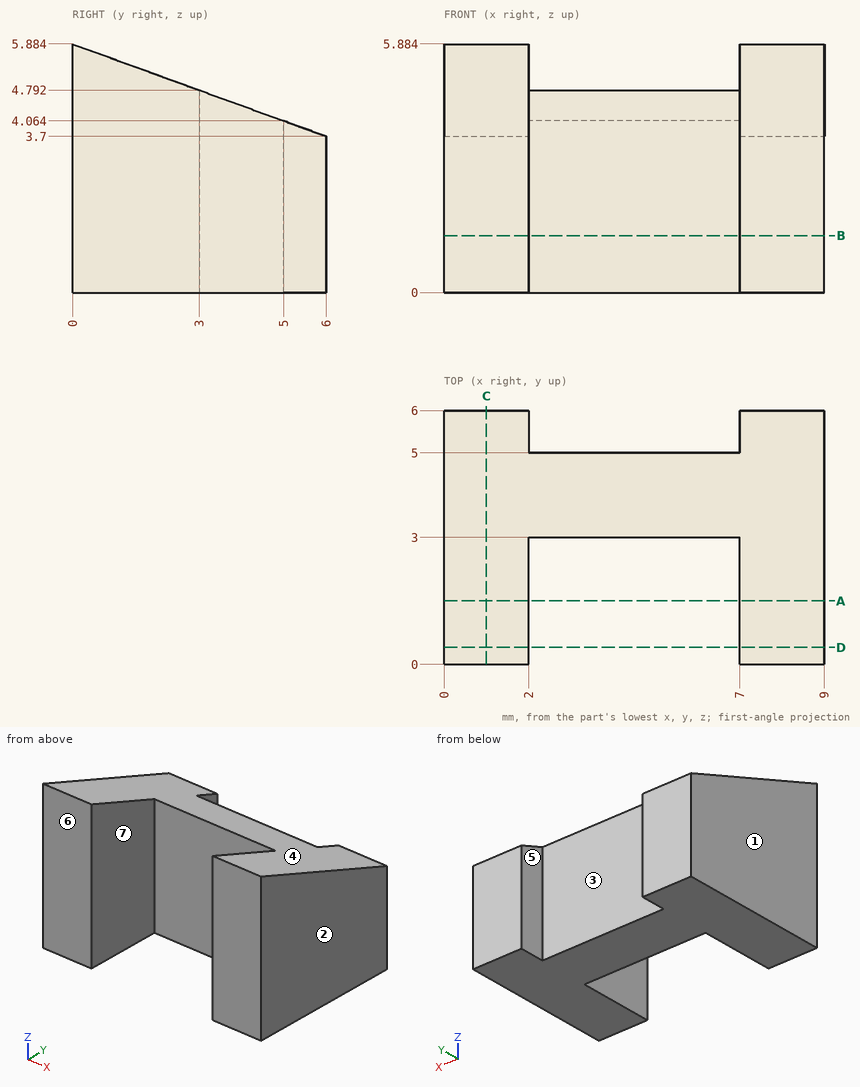
Answer from the drawing. Dimensions are ordinates in mm from the lowest x, y and z of the part. A direction names the side the tool comes from. Give positions to 0.01 mm unless a question says otherwise; leave off trailing zeros. Loops run counter-clockwise (first coordinate to the right, second up) from the corner with the lowest first, then second, coordinate; pieces in that order, holes last.
Item 1: A tool of negligible diameter and unlimited length cuts with its end or side. For the marked faces 5, 6 and 7, from which of +Z, -Z, +X, -X, +Y, -Y can it reach the whole face along a straight path? Write none if from no direction.
Derived:
face 5: +Z, -Z, +Y
face 6: +Z, -Z, +X, -X, -Y
face 7: +Z, -Z, -Y
Item 2: A cutting plane is placed at C-C (x = 1). Give the vertices of the cut face in (y, z).
Derived:
outline: (0, 0) - (6, 0) - (6, 3.7) - (0, 5.88) - close
Item 3: Determine the mould class of the marked faces 1, 2, 3 and 4 for opening direction X: +X half, -X half, draft (parallel to the pull), parting line (faces both ways), or undercut.
Derived:
face 1: -X half
face 2: +X half
face 3: undercut
face 4: draft
Item 4: A cutting plane is placed at D-D (y = 0.4). Give the vertices of the cut face in (x, z).
Derived:
outline: (0, 0) - (2, 0) - (2, 5.74) - (0, 5.74) - close; (7, 0) - (9, 0) - (9, 5.74) - (7, 5.74) - close
Item 5: A cutting plane is placed at B-B (z = 1.35). Give the vertices of the cut face in (x, y).
Derived:
outline: (0, 0) - (2, 0) - (2, 3) - (7, 3) - (7, 0) - (9, 0) - (9, 6) - (7, 6) - (7, 5) - (2, 5) - (2, 6) - (0, 6) - close
Item 6: Find the intervals of material crossed by line 1 along X through (y, z) = (1.2, 2.7); line 2 along Y through (x, z) = (5, 0.7); line 3 along Z through (x, y) = (1, 5), in increasing order.
Derived:
line 1: x = 0 to 2, 7 to 9
line 2: y = 3 to 5
line 3: z = 0 to 4.06
Item 7: Each of these flat-tipped pins is pushed along its axis until it touches: pin 1 Ø1.5 at (x, y) = (2, 4.5) entering from +Z; pin 2 Ø3 at (x, y) = (5.5, 3) entering from -Z; pin 3 Ø2.5 at (x, z) = (5, 1.5) entering from -Y; pin 4 Ø1.5 at (x, y) = (4.5, 2.5) entering from +Z. Where does it stop, or does it pass through?
Derived:
pin 1: stops at z = 4.52
pin 2: stops at z = 0
pin 3: stops at y = 3
pin 4: stops at z = 4.79
Item 8: A cutting plane is placed at A-A (y = 1.5). Give the vertices of the cut face in (x, z).
Derived:
outline: (0, 0) - (2, 0) - (2, 5.34) - (0, 5.34) - close; (7, 0) - (9, 0) - (9, 5.34) - (7, 5.34) - close
